Part model, mm, in its own coordinate system. Give positions to 0.01 mm unless a question says otherwise; leave off trailing zeros. Loops run counter-clockwise (first coordinate to the right, second up) from the corner with the lowest first, then second, coordinate; pieces in that order, holes last. Notation, with made-up numbers: (-12.5, 79) -> (-7.5, 79) arc R14 cw to (-7.5, 98) -> close; hole circle Ø8 at (-32, 80). An arc over 180 degrees is marked (long way). One line per question, with ' | ' between items.
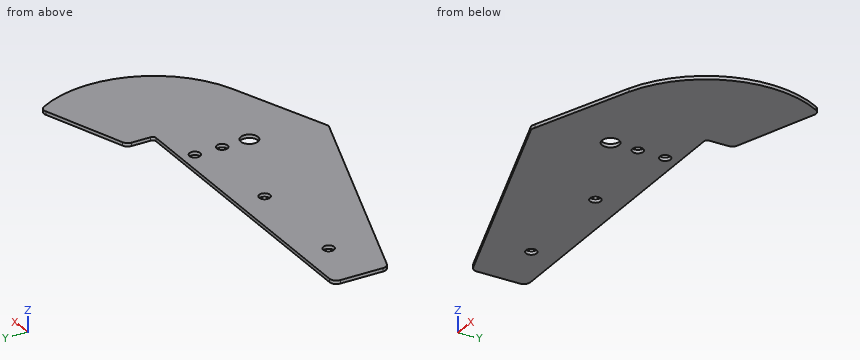
Autodesk Inventor part; units mm, degrees
ref_plane "YZ Plane" through (0, 0, 0) normal (1, 0, 0) x (0, 1, 0)
ref_plane "XZ Plane" through (0, 0, 0) normal (0, 1, 0) x (-1, 0, 0)
ref_plane "XY Plane" through (0, 0, 0) normal (0, 0, 1) x (1, 0, 0)
sketch "Sketch1" plane through (0, 0, 0) normal (0, 0, 1) x (1, 0, 0)
  spline S0 degree 3 poles (57.6456, -40.773) (58.3081, -40.9936) (59.0965, -41.3227) (60.2711, -40.8533) (60.9829, -40.5929) knots 0 0 0 0 0.471955 1 1 1 1
  line L0 (57.6456, -40.773) -> (58.3081, -40.9936) construction
  line L1 (58.3081, -40.9936) -> (59.0965, -41.3227) construction
  line L2 (59.0965, -41.3227) -> (60.2711, -40.8533) construction
  line L3 (60.2711, -40.8533) -> (60.9829, -40.5929) construction
  circle A0 centre (65.4964, 17.3655) radius 2.54
  circle A1 centre (65.4964, 4.6655) radius 2.54
  circle A2 centre (65.4964, -8.0345) radius 4
  circle A3 centre (21.0464, 11.0155) radius 2.54
  arc A4 (106.077, -23.4013) -> (131.0436, 49.1793) centre (87.0864, 23.7155) ccw
  line L4 (87.0864, 25.303) -> (87.0864, 34.1689)
  line L5 (89.2051, 37.163) -> (127.2399, 50.5819)
  circle A5 centre (-29.7536, 11.0155) radius 2.54
  line L6 (-51.9786, 23.7155) -> (85.4989, 23.7155)
  line L7 (60.9829, -40.5929) -> (106.077, -23.4013)
  line L8 (-55.1536, 20.5405) -> (-55.1536, 0.5755)
  line L9 (-53.0182, -2.4244) -> (57.6456, -40.773)
  arc A6 (-51.9786, 23.7155) -> (-55.1536, 20.5405) centre (-51.9786, 20.5405) ccw
  arc A7 (-55.1536, 0.5755) -> (-53.0182, -2.4244) centre (-51.9786, 0.5755) ccw
  arc A8 (131.0436, 49.1793) -> (127.2399, 50.5819) centre (128.2963, 47.5878) ccw
  arc A9 (89.2051, 37.163) -> (87.0864, 34.1689) centre (90.2614, 34.1689) ccw
  arc A10 (85.4989, 23.7155) -> (87.0864, 25.303) centre (85.4989, 25.303) ccw
  point P0 (129.6573, 51.4348)
  point P1 (129.6573, 51.4348)
  point P2 (-55.1536, 23.7155)
  point P3 (-55.1536, -1.6845)
  point P4 (60.9902, -40.5901)
  point P5 (129.6573, 51.4348)
  point P6 (87.0864, 36.4155)
  point P7 (60.9829, -40.5929)
  dimension "d2" = 3.175
  dimension "d3" = 1.5875
extrude "Extrusion1" add sketch "Sketch1" along normal blind 1.5875
properties part number "intake_sled"
1) Saw through at B-B (y = -20). Give the cut face in (x, z).
Found:
outline: (-2.3, 0) -> (112.96, 0) -> (112.96, 1.59) -> (-2.3, 1.59) -> close
2) Pin check, flat tips, straight feed: P1, Ø4.5, axis at x = -29.75, y = 11.02, coming from the -Z side; P2, Ø1.5, axis at x = -15.5, y = -8.5, coming from the -Z side; P3, Ø0.5, axis at y = 30, z = 0.5, coming from the -X side. Stop position of each tip, or through.
Found:
P1: through | P2: z = 0 | P3: x = 87.09
3) Drill centre lines: line 1 (X direction, y = 11, z = 1.2); line 2 (X direction, y = 10.5, z = 1.1); line 3 (X direction, y = 4.5, z = 1.3). Where is each one in solid material? Low to high.
Found:
line 1: -55.15 to -32.29, -27.21 to 18.51, 23.59 to 136.27 | line 2: -55.15 to -32.24, -27.27 to 18.56, 23.53 to 136.14 | line 3: -55.15 to 62.96, 68.03 to 134.11
4) Saw through at C-C (x = 51). Give the cut face in (y, z), and give its area (3 significant figures).
Found:
outline: (-38.47, 0) -> (23.72, 0) -> (23.72, 1.59) -> (-38.47, 1.59) -> close | area: 98.7 mm2
5) Saw through at A-A (z = 1.1). State how many separate pieces and enclosed holes the cut face has, and give its area (3 significant figures).
Found:
separate pieces: 1 | enclosed holes: 5 | area: 9,760 mm2
